from build123d import *

# Parameters (mm, degrees)
SKETCH1_R               = 4.7625
BOSS_EXTRUDE1_DEPTH     = 4.7625
SKETCH1_3_W             = 14
SKETCH1_3_H             = 22
SKETCH1_3_R             = 4.7625
BOSS_EXTRUDE2_DEPTH     = 3
FILLET1_R               = 2
SKETCH2_R               = 0.396875
SKETCH2_R_2             = 1
CUT_EXTRUDE1_DEPTH      = 17.56465552
CUT_EXTRUDE1_DEPTH_BACK = 17.56465552


with BuildPart() as part:
    # Sketch1 → Boss-Extrude1 (new body)
    with BuildSketch(Plane.XY):
        with Locations(Location((0, 0, 0), (0, 0, 180))):
            Circle(SKETCH1_R)
    extrude(amount=BOSS_EXTRUDE1_DEPTH)

    # Sketch1_3 → Boss-Extrude2 (add)
    with BuildSketch(Plane.XY):
        with Locations((0, -3.2375)):
            Rectangle(SKETCH1_3_W, SKETCH1_3_H)
        with Locations(Location((0, 0, 0), (0, 0, 180))):
            Circle(SKETCH1_3_R, mode=Mode.SUBTRACT)
        with Locations(Location((0, 0, 0), (0, 0, 180))):
            Circle(SKETCH1_3_R)
    extrude(amount=-BOSS_EXTRUDE2_DEPTH)

    # Fillet1
    fillet1_edges = [part.edges().sort_by_distance(p)[0] for p in [
        (7, -14.2375, -1.5),
        (-7, -14.2375, -1.5),
        (-7, 7.7625, -1.5),
        (7, 7.7625, -1.5),
    ]]
    fillet(fillet1_edges, radius=FILLET1_R)

    # Sketch2 → Cut-Extrude1 (cut, two sides)
    with BuildSketch(Plane.XY) as cut_extrude1_sk:
        with Locations((0, -12.7375)):
            Circle(SKETCH2_R)
        with Locations((2.5, -12.7375)):
            Circle(SKETCH2_R)
        with Locations((-2.5, -12.7375)):
            Circle(SKETCH2_R)
        with Locations((-4.4125, 5.175)):
            Circle(SKETCH2_R_2)
        with Locations((4.4125, 5.175)):
            Circle(SKETCH2_R_2)
    extrude(amount=CUT_EXTRUDE1_DEPTH, mode=Mode.SUBTRACT)
    extrude(cut_extrude1_sk.sketch, amount=-CUT_EXTRUDE1_DEPTH_BACK, mode=Mode.SUBTRACT)


solid = part.part
Part model, mm, in its own coordinate system. A direction names the side the tool comes from. Coordinates: 2 decimals unless noted, no trailing zeros. Loops run counter-clockwise (first coordinate to the right, second up) from the corner with the lowest first, then second, coordinate; pieces in that order, holes last. Notation, with made-up numbers: M 23.5,85 L 76.5,85 A12 cw 76.5,108 Z; hole C 58.5,56 d7. An arc over 180 degrees is marked long. Use a Markdown table: item, result. Add a question column.
Q1. Cut at A-A (x = 0). Write the cut outline in (y, z), and give its area (3 significant figures).
Q2. Which spindle directions (+Z, -Z, +X, -X, +Y, -Y) get a long thin tool onto all of the face, cutting with end or side? Do faces 4 (the cylindrical face through (1.03, 4.65, 2.35)), 5 (the cylindrical face through (-6.43, 7.16, -1.52)). Say none if no direction does.
Q3. Cut at C-C (z = 1.25). Write the cut outline in (x, y) (1 decimal), and give its area (3 significant figures).
Q4. Probe L1, parallel to Y at x = -2.5, z = -1.3; L2, parallel to Z at x = 5.5, y = 1; L3, parallel to Y at x = 0, z = 1.25. List the from-to ranges inside material, lowest first.
Q5. Cut at D-D (x = -2.5). Write the cut outline in (y, z).
Q6. Pin check, flat tips, straight feed: P1, Ø1, axis at x = -2, y = -11, coming from the +Z side; P2, Ø1.5, axis at x = 0.5, z = 2.5, coming from the -Y side. Stop position of each tip, or through.
Q7. Cut at B-B (y = 0). Write the cut outline in (x, z).
Q8. Mould opens along Y. For faces 1 (the flat face through (0, -6, 0)), 2 (the cylindrical face through (-6.43, -13.636, -1.521)), 3 (the cylindrical face through (-3.875, 6.018, -1.479)) say: +Y half, -Y half, draft (parallel to the pull), parting line (faces both ways), or undercut.
Worked out:
| question | item | result |
|---|---|---|
| 1 | outline | M -14.24,-3 L -13.13,-3 L -13.13,0 L -14.24,0 Z; M -12.34,-3 L 7.76,-3 L 7.76,0 L 4.76,0 L 4.76,4.76 L -4.76,4.76 L -4.76,0 L -12.34,0 Z |
| 1 | area | 109 mm2 |
| 2 | face 4 | +Z |
| 2 | face 5 | +Z, -Z, -X, +Y |
| 3 | outline | C 0,0 d9.5 |
| 3 | area | 71.3 mm2 |
| 4 | L1 | y = -14.24 to -13.13, -12.34 to 7.76 |
| 4 | L2 | z = -3 to 0 |
| 4 | L3 | y = -4.76 to 4.76 |
| 5 | outline | M -14.24,-3 L -13.13,-3 L -13.13,0 L -14.24,0 Z; M -12.34,-3 L 7.76,-3 L 7.76,0 L 4.05,0 L 4.05,4.76 L -4.05,4.76 L -4.05,0 L -12.34,0 Z |
| 6 | P1 | stops at z = 0 |
| 6 | P2 | stops at y = -4.76 |
| 7 | outline | M -7,-3 L 7,-3 L 7,0 L 4.76,0 L 4.76,4.76 L -4.76,4.76 L -4.76,0 L -7,0 Z |
| 8 | face 1 | draft |
| 8 | face 2 | -Y half |
| 8 | face 3 | undercut |
